The listing builds one solid part. Answer for the finished solid, in the listing's coordinates (mm). Face numbers are marked on the shaded views. Give positions to 0.01 mm unless a question says otherwise; leave off trailing zeros. Loops run counter-clockwise (first coordinate to the right, second up) from the corner with the lowest first, then second, coordinate; pieces in that order, holes last. Notation, with made-up numbers: (82.5, -21) - (134.5, -21) arc R10 ccw to (134.5, -7) - close; hole circle Ø1 at (89.5, 0). An arc over 180 degrees is marked (long way). Write each question's results on one line, items separated by ' | '.
from build123d import *

# Parameters (mm, degrees)
SKETCH1_R           = 1
SKETCH1_R_2         = 5
BOSS_EXTRUDE1_DEPTH = 4


with BuildPart() as part:
    # Sketch1 → Boss-Extrude1 (new body)
    with BuildSketch(Plane.XY):
        with BuildLine():
            Line((-15, -7.896321871), (-9.819449375, 18.995347754))
            ThreePointArc((-9.819449375, 18.995347754), (0, 27.103678129), (9.819449375, 18.995347754))
            Line((9.819449375, 18.995347754), (15, -7.896321871))
            Line((15, -7.896321871), (15, -32.896321871))
            Line((15, -32.896321871), (-15, -32.896321871))
            Line((-15, -32.896321871), (-15, -7.896321871))
        make_face()
        with Locations((0, 24.103678129)):
            Circle(SKETCH1_R, mode=Mode.SUBTRACT)
        with Locations((4.949747468, 22.053425597)):
            Circle(SKETCH1_R, mode=Mode.SUBTRACT)
        with Locations((7, 17.103678129)):
            Circle(SKETCH1_R, mode=Mode.SUBTRACT)
        with Locations((4.949747468, 12.153930661)):
            Circle(SKETCH1_R, mode=Mode.SUBTRACT)
        with Locations((0, 10.103678129)):
            Circle(SKETCH1_R, mode=Mode.SUBTRACT)
        with Locations((-4.949747468, 12.153930661)):
            Circle(SKETCH1_R, mode=Mode.SUBTRACT)
        with Locations((-7, 17.103678129)):
            Circle(SKETCH1_R, mode=Mode.SUBTRACT)
        with Locations((-4.949747468, 22.053425597)):
            Circle(SKETCH1_R, mode=Mode.SUBTRACT)
        with Locations((0, 17.103678129)):
            Circle(SKETCH1_R_2, mode=Mode.SUBTRACT)
    extrude(amount=BOSS_EXTRUDE1_DEPTH)


solid = part.part
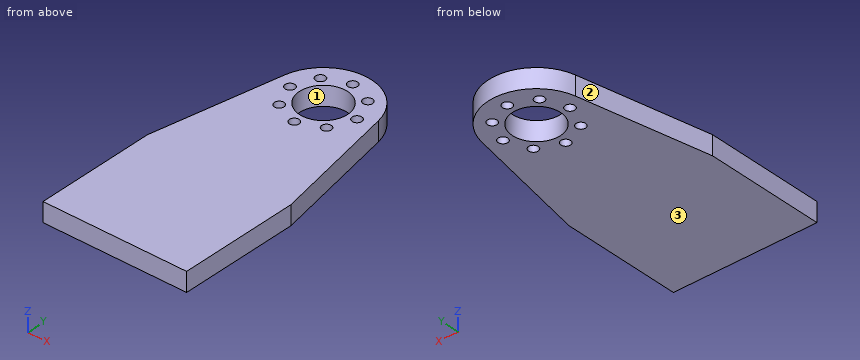
Item 1: A flat-ended cylindrical pin translates along its axis: P1, Ø1.6, axis at x = 0, y = 10.1, coming from the +Z side. Find the tip coordinate at first contact, or state that the pin passes through.
Values found:
P1: passes through
Item 2: A cutting plane is placed at B-B, the plane z = 3.3. Count the separate pieces of the cut face and the enclosed holes in it, plus the area to 3 significant figures.
Values found:
separate pieces: 1 | enclosed holes: 9 | area: 1,430 mm²
Item 3: For a pull along X with two mould halves and no side action, classify the marked faces 1, 2 and 3 as released by +X, released by -X, zero draft, split by the parting line, or undercut.
Values found:
face 1: undercut | face 2: released by -X | face 3: zero draft
Item 4: A cutting plane is placed at D-D, the plane y = 6.5. Determine the outline of the cut face in (x, z), plus the area to 3 significant figures.
Values found:
outline: (-12.23, 0) - (12.23, 0) - (12.23, 4) - (-12.23, 4) - close | area: 97.8 mm²
Item 5: A cutting plane is placed at A-A, the plane x = 0. Determine the outline of the cut face in (y, z), plus the area to 3 significant figures.
Values found:
outline: (-32.9, 0) - (9.1, 0) - (9.1, 4) - (-32.9, 4) - close; (11.1, 0) - (12.1, 0) - (12.1, 4) - (11.1, 4) - close; (22.1, 0) - (23.1, 0) - (23.1, 4) - (22.1, 4) - close; (25.1, 0) - (27.1, 0) - (27.1, 4) - (25.1, 4) - close | area: 184 mm²
Item 6: A cutting plane is placed at C-C, the plane x = -7. Determine the outline of the cut face in (y, z).
Values found:
outline: (-32.9, 0) - (16.1, 0) - (16.1, 4) - (-32.9, 4) - close; (18.1, 0) - (24.25, 0) - (24.25, 4) - (18.1, 4) - close
Item 7: Find the intervals of material crossed by line 1 along Y through (x, z) = (0, 3.1); line 2 along X through (y, z) = (13, 3.5); line 3 along X through (y, z) = (12, 3.7), in increasing order. Write a range as [from, to].
Values found:
line 1: y = [-32.9, 9.1], [11.1, 12.1], [22.1, 23.1], [25.1, 27.1] | line 2: x = [-10.97, -5.48], [-4.42, -2.86], [2.86, 4.42], [5.48, 10.97] | line 3: x = [-11.17, -5.94], [-3.96, 3.96], [5.94, 11.17]
